Geometry check sheet. Reference: drawing and pictorial views, mm from the part's lowest x, y, z. A direction names the side the tool comes from. Coordinates: 2 decimals unless noted, no trailing zeros. Loops run counter-clockwise (first coordinate to the right, second up) from the corner with the lowest first, then second, coordinate; pieces in that order, holes last. Notation, with made-up numbers: (-36, 23) - (5, 23) arc R13 cw to (5, 43) - close; hole circle Ø5 at (4, 65.5). An arc over 180 degrees is marked (long way). Use a Markdown table: item, result. Add a question column.
1) Sectioned sample at C-C, the plane z = 6. Enter the section's corners in (x, y).
2) Tool access check on the marked faces 5 and 6. Record the directions out of +Z, -Z, +X, -X, +Y, -Y that give a thin tool (end or side, any length) a straight path to the whole face; none if there is none.
3) Thickness scan on line 1 (X direction, y = 41, z = 14.75); line 2 (Y direction, x = 45, z = 11); line 3 (Y direction, x = 10, z = 6). Record the ranges inside material, lowest first.
4) Sectioned sample at D-D, the plane y = 66.5. Enter the section's corners in (x, z).
5) Sectioned sample at A-A, the plane x = 50. Enter the section's corners in (y, z).
6) Sectioned sample at B-B, the plane y = 90. Enter the section's corners in (x, z), then the cut area to 3 significant figures.
7) Go/stop test with flat-tipped pins: P1, Ø3, axis at x = 92.5, z = 7, coming from the -Y side; P2, Ø4, axis at y = 16, z = 10.5, coming from the +X side; P3, Ø2, axis at x = 73.5, y = 66.5, coming from the +Z side; P4, Ø2.5, axis at x = 10, y = 10, coming from the -Z side. Record where each tip stops, or that it passes through.
8) Draft check along Y on the marked faces 1, 2, 3 and 4. Enter one of: pulls with the +Y half, pulls with the -Y half, needs draft (parallel to the pull), parting line crosses it, or undercut.
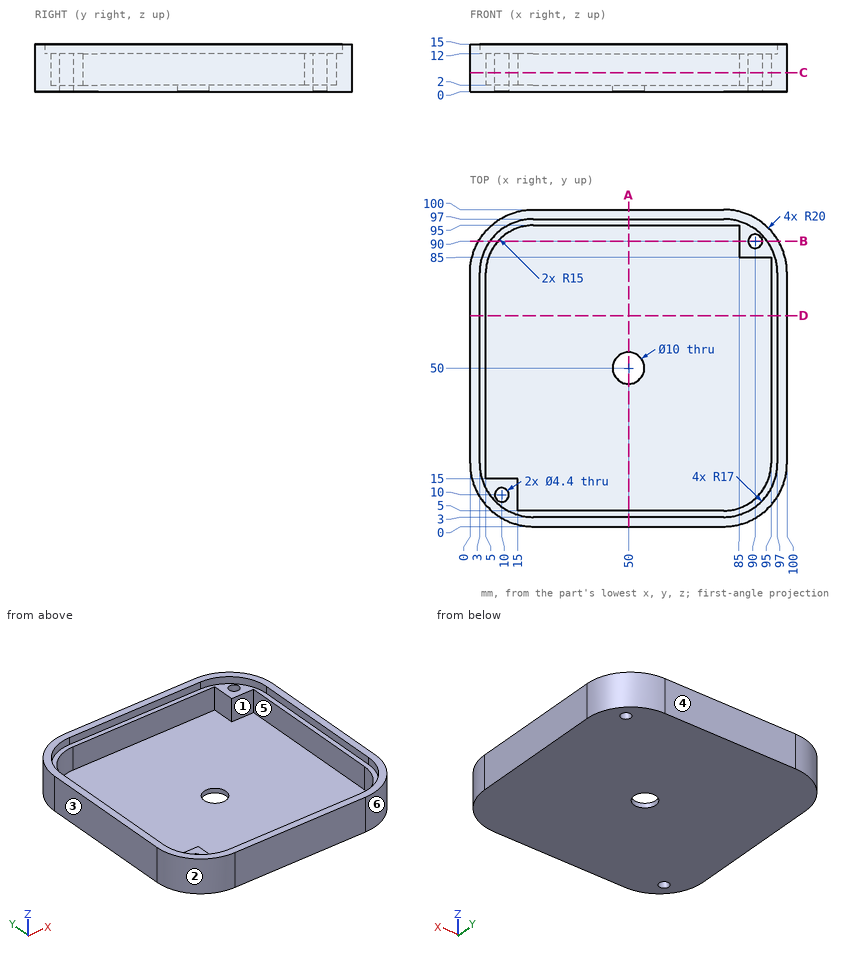
Solved:
| question | item | result |
|---|---|---|
| 1 | outline | (0, 20) arc R20 ccw to (20, 0) - (80, 0) arc R20 ccw to (100, 20) - (100, 80) arc R20 ccw to (80, 100) - (20, 100) arc R20 ccw to (0, 80) - close; hole (5, 15) - (15, 15) - (15, 5) - (80, 5) arc R15 ccw to (95, 20) - (95, 85) - (85, 85) - (85, 95) - (20, 95) arc R15 ccw to (5, 80) - close; hole circle Ø4.4 at (10, 10); hole circle Ø4.4 at (90, 90) |
| 2 | face 5 | +Z |
| 2 | face 6 | +Z, -Z, +X, -Y |
| 3 | line 1 | x = 0 to 3, 97 to 100 |
| 3 | line 2 | y = 0 to 5, 95 to 100 |
| 3 | line 3 | y = 2.68 to 7.8, 12.2 to 15, 91.18 to 97.32 |
| 4 | outline | (0, 0) - (100, 0) - (100, 15) - (97, 15) - (97, 12) - (95, 12) - (95, 2) - (5, 2) - (5, 12) - (3, 12) - (3, 15) - (0, 15) - close |
| 5 | outline | (0, 0) - (45, 0) - (45, 2) - (5, 2) - (5, 12) - (3, 12) - (3, 15) - (0, 15) - close; (55, 0) - (100, 0) - (100, 15) - (97, 15) - (97, 12) - (95, 12) - (95, 2) - (55, 2) - close |
| 6 | outline | (2.68, 0) - (87.8, 0) - (87.8, 12) - (85, 12) - (85, 2) - (8.82, 2) - (8.82, 12) - (6.25, 12) - (6.25, 15) - (2.68, 15) - close; (92.2, 0) - (97.32, 0) - (97.32, 15) - (93.75, 15) - (93.75, 12) - (92.2, 12) - close |
| 6 | area | 343 mm2 |
| 7 | P1 | stops at y = 3.3 |
| 7 | P2 | stops at x = 99.9 |
| 7 | P3 | stops at z = 2 |
| 7 | P4 | passes through |
| 8 | face 1 | undercut |
| 8 | face 2 | pulls with the -Y half |
| 8 | face 3 | needs draft |
| 8 | face 4 | pulls with the +Y half |
